Geometry: see drawing. Coordinates: mm, zero at the bounding-box minimum. A direction names the side the tool comes from. Give positions to 0.01 mm unless a question says otherwise; leave off trailing zeros. Order: outer loops, then holes, each group sorted by start corner. A loop starts at its lowest first (then second) coordinate and runs counter-clockwise, first axis right, second up. Notation, with made-up numbers: (44, 35) - (76, 35) arc R21 cw to (76, 41) - close; hole circle Ø4 at (75.5, -33.75). An arc over 180 degrees is marked (long way). Put each result on its own line as item: value. Start each with the question number.
1. Section A-A on x = 17.25. Return the cut outline in (y, z), plus the area to 3 significant figures.
2. Ray query, line 1 along Y through (x, z) = (4.75, 3); line 2 along Y through (x, z) = (8, 17.5); line 3 along Z through (x, y) = (18.5, 9.75). Return the intervals inside material, ascending. Write a range as from..to.
3. Set-up query: the marked faces 5 and 6. Return all of +Z, -Z, +X, -X, +Y, -Y with unobstructed straight access to the full face (end or side cutting, diameter ignored); none if empty.
4. Section D-D on z = 32. Return the cut outline in (x, y).
5. Mould query, pull axis Y, two halves, no side actions, for the marked faces 1, 2, 3 and 4. Classes: pulls with the +Y half, pulls with the -Y half, needs draft (parallel to the pull), parting line crosses it, or undercut.
6. Section B-B on z = 9. Return the cut outline in (x, y).
7. Section C-C on y = 4. Return the cut outline in (x, z) (3 decimals).
8. First-contact query: P1, Ø10, axis at y = 12.5, z = 19.5, coming from the +X side; P2, Ø10, axis at x = 13, z = 44, coming from the -Y side; P3, Ø2, axis at x = 9.5, y = 14, coming from the +Z side; P4, Ø1.6, axis at x = 9, z = 16, coming from the -Y side. Flat tips, straight axial feed; report the tip coordinate or a pass-through.
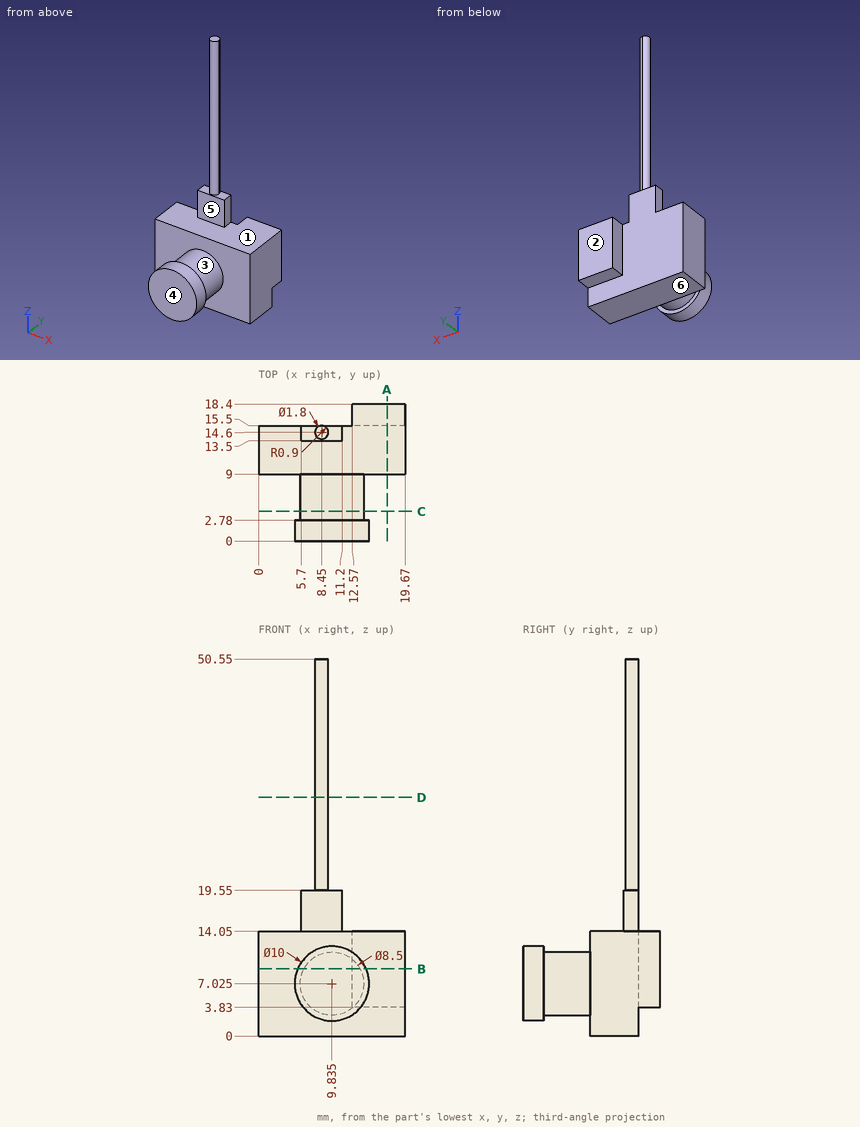
Resolved:
1. outline: (9, 0) - (15.5, 0) - (15.5, 3.83) - (18.4, 3.83) - (18.4, 14.05) - (9, 14.05) - close
1. area: 121 mm^2
2. line 1: 9..15.5
2. line 2: 13.5..15.5
2. line 3: 0..14.05
3. face 5: +Z, +X, -X, -Y
3. face 6: -Z, +X, -X, +Y, -Y
4. outline: circle Ø1.8 at (8.45, 14.6)
5. face 1: needs draft
5. face 2: pulls with the +Y half
5. face 3: undercut
5. face 4: pulls with the -Y half
6. outline: (0, 9) - (6.07, 9) - (6.07, 2.78) - (5.24, 2.78) - (5.24, 0) - (14.43, 0) - (14.43, 2.78) - (13.6, 2.78) - (13.6, 9) - (19.67, 9) - (19.67, 18.4) - (12.57, 18.4) - (12.57, 15.5) - (0, 15.5) - close
7. outline: circle Ø8.5 at (9.835, 7.025)
8. P1: x = 11.2
8. P2: y = 13.7
8. P3: z = 50.55
8. P4: y = 13.5
